Source: CAD feature listing. Evaluate the final solid. Frame: model axes, mm. A direction names the side the tool comes from. Round coordinates to 2 decimals unless told otherwise and drop trailing zeros. Loops run counter-clockwise (first coordinate to the right, second up) from the corner with the lowest first, then second, coordinate; pieces in that order, holes last. Notation, with made-up numbers: M 69,62.25 L 117,62.25 A18 cw 117,69.25 Z; hole C 13.5,46.5 d3. An arc over 180 degrees is marked long. Answer as a JSON object with one key per item and string values.
Autodesk Inventor part; units mm, degrees
ref_plane "YZ Plane" through (0, 0, 0) normal (1, 0, 0) x (0, 1, 0)
ref_plane "XZ Plane" through (0, 0, 0) normal (0, 1, 0) x (-1, 0, 0)
ref_plane "XY Plane" through (0, 0, 0) normal (0, 0, 1) x (1, 0, 0)
sketch "Sketch5" plane through (0, 0, 0) normal (0, 0, 1) x (1, 0, 0)
  line L0 (0, 0) -> (0, 27)
  line L1 (170, 0) -> (170, 27)
  line L2 (170, 27) -> (204, 27)
  line L3 (204, 27) -> (204, 2)
  line L4 (204, 2) -> (209, 2)
  line L5 (209, 2) -> (209, 0)
  line L6 (209, 0) -> (170, 0)
  point P0 (189.5, 0)
  dimension "d16" = 340
  dimension "d17" = 408
  dimension "d19" = 25
  dimension "d20" = 2
  dimension "d21" = 5
revolve "Revolution1" add sketch "Sketch5" angle 360 about axis through (0, 0, 0) along (0, 1, 0)
sketch "Sketch6" plane through (0, 27, 0) normal (0, 1, 0) x (1, 0, 0)
  circle A0 centre (0, 0) radius 184
  line L0 (0, 0) -> (-70.4138, 169.9938)
  line L1 (0, 0) -> (0, 184)
  dimension "d23" = 368
  dimension "d34" = 22.5
hole "Hole1" at (-70.4138, 27, -169.9938) direction (0, -1, 0) diameter 11 end through all counterbore diameter 20 counterbore depth 10
pattern_circular "Circular Pattern2" count 8 over 360 about axis through (0, -10, 0) along (0, 1, 0) of "Hole1"
sketch "Sketch7" plane through (0, 0, 0) normal (0, 1, 0) x (-1, 0, 0)
  circle A0 centre (0, 0) radius 209
  circle A1 centre (0, 0) radius 170
  line L0 (0, 0) -> (0, -209)
  line L1 (0, 0) -> (-209, 0)
  point P0 (-170, 0)
  point P1 (0, -170)
  dimension "d35" = 90
extrude "Extrusion5" [suppressed]
equation "\"d29\" = Thickness"
properties part number "DMF 01 33 Барабан Опорное кольцо КОРМА v2.5"
Item 1: Line query: probe 1 along Z at (x, y) = (173.5, 24.25); probe 2 along Z at (x, y) = (-5, 3); probe 3 along X at (y, z) = (6.75, -57). Output: solid intervals per line, ascending. Write a range as from..to.
Answer sheet:
{"probe 1": "z = -107.3..-79.78, -61.05..61.05, 79.78..107.3", "probe 2": "z = -203.94..-169.93, 169.93..203.94", "probe 3": "x = -195.87..-160.16, 160.16..195.87"}
Item 2: Section A-A on x = 0. Return the cut outline in (y, z).
Answer sheet:
{"outline": "M 0,-209 L 2,-209 L 2,-204 L 27,-204 L 27,-170 L 0,-170 Z; M 0,170 L 27,170 L 27,204 L 2,204 L 2,209 L 0,209 Z"}
Item 3: Section B-B on z = 0. Return the cut outline in (x, y), then the cut area to 3 significant figures.
Answer sheet:
{"outline": "M -209,0 L -170,0 L -170,27 L -204,27 L -204,2 L -209,2 Z; M 170,0 L 209,0 L 209,2 L 204,2 L 204,27 L 170,27 Z", "area": "1,860 mm²"}
Item 4: Pull-direction query (X, two-part tool) for faces 1 (the cylindrical face through (112.4, 1, 176.2)), 2 (the cylindrical face through (70.65, 8.38, -175.49)), 3 (the flat face through (200, 2, 45)); classes: pulls with the +X half, pulls with the -X half, needs draft (parallel to the pull), parting line crosses it, or undercut.
Answer sheet:
{"face 1": "parting line crosses it", "face 2": "undercut", "face 3": "needs draft"}
Item 5: Access query for faces 4 (the cylindrical face through (-44.22, 14.32, -199.15)), 5 (the cylindrical face through (-175.49, 8.38, -70.65)). Directions: +Z, -Z, +X, -X, +Y, -Y. A direction counts if a zero-diameter tool reaches every point of the face in a straight line with its end or side. Return the directions, or none.
Answer sheet:
{"face 4": "+Y", "face 5": "+Y, -Y"}
Item 6: Section C-C on y = 11.5. Give the number of separate pieces and of enclosed holes in the cut face, then the cut area to 3 significant figures.
Answer sheet:
{"separate pieces": "1", "enclosed holes": "9", "area": "39,200 mm²"}
Item 7: Contact query for flat-ended pins moving along their axis: pin 1 Ø12 at (x, z) = (70.41, -169.99) entering from -Y; pin 2 Ø1 at (x, y) = (-122.5, 23) entering from -Z; pin 3 Ø6 at (x, z) = (-72.5, -168) entering from +Y; pin 4 Ø2 at (x, y) = (-9.5, 17) entering from +Z. Output: stop coordinate, or through.
Answer sheet:
{"pin 1": "stops at y = 0", "pin 2": "stops at z = -163.5", "pin 3": "stops at y = 17", "pin 4": "stops at z = 203.82"}
